```python
from build123d import *

# Parameters (mm, degrees)
SKETCH1_W           = 629.90984
SKETCH1_H           = 147.69846
BOSS_EXTRUDE1_DEPTH = 3.175
SKETCH3_W           = 254
SKETCH3_H           = 3.175
BOSS_EXTRUDE2_DEPTH = 6.35
SKETCH4_W           = 3.175
SKETCH4_H           = 188.732840052
CUT_EXTRUDE1_DEPTH  = 3.175
SKETCH6_W           = 3.175
SKETCH6_H           = 110.773845
BOSS_EXTRUDE4_DEPTH = 3.175
SKETCH8_W           = 629.90984
SKETCH8_H           = 18.04416
BOSS_EXTRUDE5_DEPTH = 3.175
SKETCH10_W          = 38.1
SKETCH10_H          = 18.04416
SKETCH10_H_2        = 36.08832
CUT_EXTRUDE3_DEPTH  = 652.56536379
BOSS_EXTRUDE6_DEPTH = 3.175


with BuildPart() as part:
    # Sketch1 → Boss-Extrude1 (new body)
    with BuildSketch(Plane(origin=(0, 0, 0), x_dir=(1, 0, 0), z_dir=(0, 1, 0))):
        with Locations((314.95492, 73.84923)):
            Rectangle(SKETCH1_W, SKETCH1_H)
    extrude(amount=BOSS_EXTRUDE1_DEPTH)

    # Sketch3 → Boss-Extrude2 (add)
    with BuildSketch(Plane(origin=(0, 0, -147.69846), x_dir=(-1, 0, 0), z_dir=(0, 0, -1))):
        with Locations((-473.22613, 1.5875)):
            Rectangle(SKETCH3_W, SKETCH3_H)
        with Locations((-156.68371, 1.5875)):
            Rectangle(SKETCH3_W, SKETCH3_H)
    extrude(amount=BOSS_EXTRUDE2_DEPTH)

    # Sketch4 → Cut-Extrude1 (cut)
    with BuildSketch(Plane(origin=(0, 3.175, 0), x_dir=(1, 0, 0), z_dir=(0, 1, 0))):
        with Locations((314.95492, 147.69846)):
            Rectangle(SKETCH4_W, SKETCH4_H)
    extrude(amount=-CUT_EXTRUDE1_DEPTH, mode=Mode.SUBTRACT)

    # Sketch6 → Boss-Extrude4 (add)
    with BuildSketch(Plane(origin=(0, 3.175, 0), x_dir=(1, 0, 0), z_dir=(0, 1, 0))):
        with Locations((631.49734, 92.3115375)):
            Rectangle(SKETCH6_W, SKETCH6_H)
        with Locations((-1.5875, 92.3115375)):
            Rectangle(SKETCH6_W, SKETCH6_H)
    extrude(amount=-BOSS_EXTRUDE4_DEPTH)

    # Sketch8 → Boss-Extrude5 (add, through all)
    with BuildSketch(Plane(origin=(0, 3.175, 0), x_dir=(1, 0, 0), z_dir=(0, 1, 0))):
        with Locations((314.95492, -9.02208)):
            Rectangle(SKETCH8_W, SKETCH8_H)
    extrude(amount=-BOSS_EXTRUDE5_DEPTH)

    # Sketch10 → Cut-Extrude3 (cut, through all)
    with BuildSketch(Plane(origin=(0, 3.175, 0), x_dir=(1, 0, 0), z_dir=(0, 1, 0))):
        with Locations((374.1674, -9.02208)):
            Rectangle(SKETCH10_W, SKETCH10_H)
        with Locations((255.74244, -9.02208)):
            Rectangle(SKETCH10_W, SKETCH10_H)
        with Locations((566.40984, -18.04416)):
            Rectangle(SKETCH10_W, SKETCH10_H_2)
        with Locations((63.5, -18.04416)):
            Rectangle(SKETCH10_W, SKETCH10_H_2)
    extrude(amount=-CUT_EXTRUDE3_DEPTH, mode=Mode.SUBTRACT)

    # Sketch11 → Boss-Extrude6 (add, through all)
    with BuildSketch(Plane(origin=(0, 3.175, 0), x_dir=(1, 0, 0), z_dir=(0, 1, 0))):
        Polygon((92.70492, -18.04416), (92.70492, -137.42416), (537.20492, -137.42416), (537.20492, -18.04416), (393.2174, -18.04416), (393.2174, -27.06624), (355.1174, -27.06624), (355.1174, -18.04416), (274.79244, -18.04416), (274.79244, -26.95194), (236.69244, -26.95194), (236.69244, -18.04416), align=None)
    extrude(amount=-BOSS_EXTRUDE6_DEPTH)


solid = part.part
```
CAD build for the part. Positions are in the model's coordinates, mm. Give positions to 0.01 mm unless a question says otherwise; leave off trailing zeros. Order: outer loops, then holes, each group sorted by start corner. A loop starts at its lowest first (then second) coordinate and runs counter-clockwise, first axis right, second up.
(1) Saw through at C-C, the plane x = 65.5. Give the cut face in (y, z) (3 decimals), then the cut area to 3 significant figures.
(2) Saw through at A-A, the plane x = 248. Give the cut face in (y, z) (3 decimals), then the cut area to 3 significant figures.
(3) Drill centre lines: L1, parallel to X at y = 3, z = -78 (3 decimals); L2, parallel to Z at x = 88, y = 2.75; L3, parallel to X at y = 0.8, z = 90. Where is each one in solid material? Low to high.
(4) Flat gauge pins, fed straight in: pin 1 (1 mm diameter, centred on x = 12, y = 2.5, fed in from -Z); pin 2 (1.6 mm diameter, centred on y = 1.5, z = 11.5, fed in from -X); pin 3 (1 mm diameter, centred on x = -1.5, y = 1.5, fed in from +Z). Where does each tip first touch, or does it go through?
(5) Saw through at B-B, the plane z = 87. Give the cut face in (x, y) (3 decimals).
(6) Saw through at D-D, the plane y = 2.45. State how many separate pieces and enclosed holes the cut face has, then the cut area to 3 significant figures.
Results found:
1. outline: (0, -154.048) - (3.175, -154.048) - (3.175, 0) - (0, 0) - close
1. area: 489 mm2
2. outline: (0, -154.048) - (3.175, -154.048) - (3.175, 0) - (0, 0) - close; (0, 26.952) - (3.175, 26.952) - (3.175, 137.424) - (0, 137.424) - close
2. area: 840 mm2
3. L1: x = -3.175 to 313.367, 316.542 to 633.085
3. L2: z = -154.05 to 18.04
3. L3: x = 92.7 to 537.2
4. pin 1: stops at z = -147.7
4. pin 2: stops at x = 0
4. pin 3: stops at z = -36.92
5. outline: (92.705, 0) - (537.205, 0) - (537.205, 3.175) - (92.705, 3.175) - close
6. separate pieces: 1
6. enclosed holes: 2
6. area: 158,000 mm2
